Geometry: final body of the model. Coordinates: model frame, mm. Face numbers are marked on the shaded views. Coordinates: 2 decimals unless noted, no trailing zeros. Write each loop counter-clockwise with the first axis right and the second up, starting at its lowest first coordinate (ties: lowest second). Pieces come first, ordered by that corner, then holes. Notation, with made-up numbers: (74.5, -3) - (96.5, -3) arc R24 cw to (96.5, 7) - close; hole circle Ø9 at (20, 20). An arc over 180 degrees is marked (long way). Answer as a JSON object with one key per item and string values. Group by question number.
Item 1: First-contact query: pin 1 Ø3 at (x, z) = (21, 0) entering from +Y; pin 2 Ø10 at (x, z) = (-6, 1.5) entering from +Y; pin 3 Ø8 at (x, z) = (3.5, -1.5) entering from +Y. Flat tips, straight axial feed; report the tip coordinate or a pass-through.
Item 2: Mould query, pull axis X, two halves, no side actions, for the marked faces 1, 2 and 3. Classes: pulls with the +X half, pulls with the -X half, needs draft (parallel to the pull), parting line crosses it, or undercut.
Item 3: Section D-D on y = -16.5. Return loops of the section in (x, z), and give its area (3 significant figures).
Item 4: Section A-A on x = -21. Return loops of the section in (y, z), and give its area (3 significant figures).
Item 5: Section B-B on z = 0. Return loops of the section in (x, y), and give its area (3 significant figures).
Item 6: Section C-C on y = -26. Return loops of the section in (x, z).
Item 7: Line query: line 1 along Z through (x, y) = (21, -25.75); line 2 along Y through (x, z) = (16, 4.5); line 3 along X through (y, z) = (-22.5, -0.5). Output: solid intervals per line, ascending. Write a range as from..to.
```python
from build123d import *

# Parameters (mm, degrees)
EXTRUDE_1_DEPTH       = 25
HOLE_WIZARD_6_0_6_1_D = 6
HOLE_WIZARD_M4_1_D    = 3.3


with BuildPart() as part:
    # 草图1 → 凸台-拉伸1 (new, symmetric)
    with BuildSketch(Plane(origin=(0, 0, 0), x_dir=(0, 0, -1), z_dir=(1, 0, 0))):
        with BuildLine():
            Line((-15, -31), (15, -31))
            Line((15, -31), (15, -14.696938457))
            ThreePointArc((15, -14.696938457), (0, -21), (-15, -14.696938457))
            Line((-15, -14.696938457), (-15, -31))
        make_face()
    extrude(amount=EXTRUDE_1_DEPTH, both=True)

    # Ø6.0 (6) 直径孔1 (through all)
    with Locations(Plane(origin=(0, 0, -15), x_dir=(-1, 0, 0), z_dir=(0, 0, -1))):
        with Locations((-15, -26), (15, -26)):
            Hole(HOLE_WIZARD_6_0_6_1_D / 2)

    # M4 螺纹孔1 (through all)
    with Locations(Plane(origin=(0, -31, 0), x_dir=(-1, 0, 0), z_dir=(0, -1, 0))):
        with Locations((-21, 0), (21, 0)):
            Hole(HOLE_WIZARD_M4_1_D / 2)


solid = part.part
```
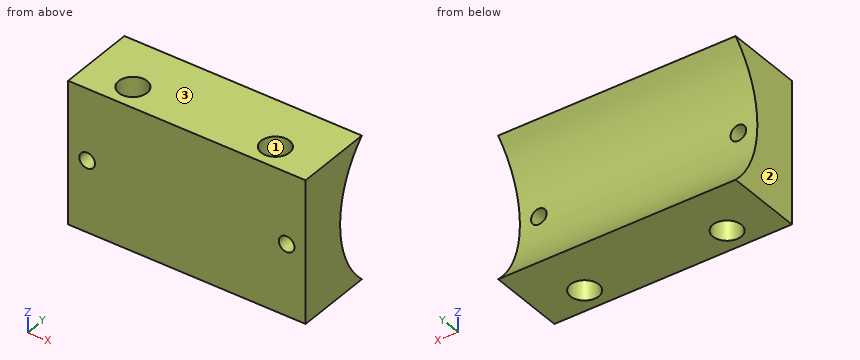
Checks:
{
 "1": {"pin 1": "through", "pin 2": "y = -19.97", "pin 3": "y = -20.27"},
 "2": {"face 1": "undercut", "face 2": "pulls with the -X half", "face 3": "needs draft"},
 "3": {"outline": "(-25, -15) - (25, -15) - (25, -12.99) - (-25, -12.99) - close; (-25, 12.99) - (25, 12.99) - (25, 15) - (-25, 15) - close", "area": "201 mm^2"},
 "4": {"outline": "(-31, -15) - (-14.7, -15) arc R21 cw to (-20.94, -1.65) - (-31, -1.65) - close; (-31, 1.65) - (-20.94, 1.65) arc R21 cw to (-14.7, 15) - (-31, 15) - close", "area": "326 mm^2"},
 "5": {"outline": "(-25, -31) - (-22.65, -31) - (-22.65, -21) - (-25, -21) - close; (-19.35, -31) - (19.35, -31) - (19.35, -21) - (-19.35, -21) - close; (22.65, -31) - (25, -31) - (25, -21) - (22.65, -21) - close; hole circle Ø6 at (-15, -26); hole circle Ø6 at (15, -26)", "area": "377 mm^2"},
 "6": {"outline": "(-25, -15) - (-18, -15) - (-18, 15) - (-25, 15) - close; (-12, -15) - (12, -15) - (12, 15) - (-12, 15) - close; (18, -15) - (25, -15) - (25, 15) - (18, 15) - close; hole circle Ø3.3 at (-21, 0); hole circle Ø3.3 at (21, 0)"},
 "7": {"line 1": "-15..-1.65, 1.65..15", "line 2": "-31..-28.83, -23.17..-20.51", "line 3": "-25..-22.57, -19.43..19.43, 22.57..25"}
}
